```python
from build123d import *

# Parameters (mm, degrees)
ESBO_O1_W                = 140
ESBO_O1_H                = 70
RESSALTO_EXTRUS_O1_DEPTH = 30
ESBO_O2_W                = 60
ESBO_O2_H                = 30
CORTE_EXTRUS_O1_DEPTH    = 31
ESBO_O3_R                = 5
CORTE_EXTRUS_O3_DEPTH    = 31


with BuildPart() as part:
    # Esboço1 → Ressalto-extrusão1 (new body)
    with BuildSketch(Plane.XY):
        Rectangle(ESBO_O1_W, ESBO_O1_H)
    extrude(amount=RESSALTO_EXTRUS_O1_DEPTH)

    # Esboço2 → Corte-extrusão1 (cut, through all)
    with BuildSketch(Plane.XY.offset(30)):
        Rectangle(ESBO_O2_W, ESBO_O2_H)
    extrude(amount=-CORTE_EXTRUS_O1_DEPTH, mode=Mode.SUBTRACT)

    # Esboço3 → Corte-extrusão3 (cut, through all)
    with BuildSketch(Plane.XY.offset(30)):
        with Locations((-58, 23)):
            Circle(ESBO_O3_R)
        with Locations((58, 23)):
            Circle(ESBO_O3_R)
        with Locations((58, -23)):
            Circle(ESBO_O3_R)
        with Locations((-58, -23)):
            Circle(ESBO_O3_R)
    extrude(amount=-CORTE_EXTRUS_O3_DEPTH, mode=Mode.SUBTRACT)


solid = part.part
```
Model file for the job. Use its own axes, mm. A direction names the side the tool comes from. Give positions to 0.01 mm unless a question says otherwise; leave off trailing zeros. Write each loop counter-clockwise with the first axis right and the second up, starting at its lowest first coordinate (ties: lowest second). Pieces come first, ordered by that corner, then holes. Notation, with made-up numbers: (39.25, -39) - (64.25, -39) arc R35 cw to (64.25, -4) - close; hole circle Ø6 at (-14, 9.5). An arc over 180 degrees is marked (long way). One line per question, with ' | ' between items. Start each with the question number.
(1) 3-axis set-ups, long thin cutter, end or side, ignore diameter. For faces 1 (the face through (-1, 16, 30)), 2 (the face through (0, 15, 15)): which of +Z, -Z, +X, -X, +Y, -Y reach the whole face in a straight line?
(2) Slice it at B-B on y = -3.5. Write the cut outline in (x, z).
(3) Slice it at C-C on x = -58. Write the cut outline in (y, z).
(4) Slice it at A-A on x = 28.5. Write the cut outline in (y, z).
(5) Two-plate mould, pull along X, no slides. Class faces 3 (the face through (56.92, -27.88, 15.21)), 4 (the face through (30, 0, 15)), 5 (the face through (70, 0, 15)), 6 (the face through (-1, 35, 15)): +X half, -X half, draft (parallel to the pull), parting line (faces both ways), or undercut.
(6) Pin check, flat tips, straight feed: P1, Ø13, axis at x = -58, y = 23, coming from the +Z side; P2, Ø8, axis at x = -58, y = -23, coming from the -Z side. Stop position of each tip, or through.
(7) Slice it at D-D on y = 23. Write the cut outline in (x, z), plus the area to 3 significant figures.
(8) Wall check: line 1 along Y through (x, z) = (58, 8.75); line 2 along Y through (x, z) = (-16, 28.75); line 3 along Y through (x, z) = (-62.5, 28). Give the ranges that are in metal, low to high. Write a range as from..to.
Results below:
1) face 1: +Z, +X, -X, +Y, -Y | face 2: +Z, -Z
2) outline: (-70, 0) - (-30, 0) - (-30, 30) - (-70, 30) - close; (30, 0) - (70, 0) - (70, 30) - (30, 30) - close
3) outline: (-35, 0) - (-28, 0) - (-28, 30) - (-35, 30) - close; (-18, 0) - (18, 0) - (18, 30) - (-18, 30) - close; (28, 0) - (35, 0) - (35, 30) - (28, 30) - close
4) outline: (-35, 0) - (-15, 0) - (-15, 30) - (-35, 30) - close; (15, 0) - (35, 0) - (35, 30) - (15, 30) - close
5) face 3: undercut | face 4: undercut | face 5: +X half | face 6: draft
6) P1: z = 30 | P2: through
7) outline: (-70, 0) - (-63, 0) - (-63, 30) - (-70, 30) - close; (-53, 0) - (53, 0) - (53, 30) - (-53, 30) - close; (63, 0) - (70, 0) - (70, 30) - (63, 30) - close | area: 3,600 mm^2
8) line 1: -35..-28, -18..18, 28..35 | line 2: -35..-15, 15..35 | line 3: -35..-25.18, -20.82..20.82, 25.18..35
